CAD build for the part. Positions are in the model's coordinates, mm. A direction names the side the tool comes from. Give positions to 0.01 mm unless a question says otherwise; leave off trailing zeros. Loops run counter-clockwise (first coordinate to the right, second up) from the corner with the lowest first, then second, coordinate; pieces in that order, holes last. Notation, with made-up numbers: M 77.25,6.25 L 107.25,6.25 A17 cw 107.25,29.25 Z; hole C -12.75,40 d1. An arc over 180 degrees is marked long. Answer as CSV lines item,"result".
from build123d import *

# Parameters (mm, degrees)
BOSS_EXTRUDE1_DEPTH                               = 12.7
SKETCH2_R                                         = 4.1
CUT_EXTRUDE1_DEPTH                                = 51.982782527
CBORE_FOR_M5_HEX_HEAD_BOLT1_D                     = 2.5
CBORE_FOR_M5_HEX_HEAD_BOLT1_DEPTH                 = 18
CBORE_FOR_M5_HEX_HEAD_BOLT1_CBORE_D               = 5.6
CBORE_FOR_M5_HEX_HEAD_BOLT1_CBORE_DEPTH           = 2.7
CBORE_FOR_M5_HEX_HEAD_BOLT1_TIP                   = 0.751075774
CBORE_FOR_M5_HEX_HEAD_BOLT1_ON_FACE_2_D           = 2.5
CBORE_FOR_M5_HEX_HEAD_BOLT1_ON_FACE_2_DEPTH       = 18
CBORE_FOR_M5_HEX_HEAD_BOLT1_ON_FACE_2_CBORE_D     = 5.6
CBORE_FOR_M5_HEX_HEAD_BOLT1_ON_FACE_2_CBORE_DEPTH = 2.7
CBORE_FOR_M5_HEX_HEAD_BOLT1_ON_FACE_2_TIP         = 0.751075774


with BuildPart() as part:
    # Sketch1 → Boss-Extrude1 (new body)
    with BuildSketch(Plane(origin=(0, 0, 0), x_dir=(1, 0, 0), z_dir=(0, 1, 0))):
        with BuildLine():
            Line((-0.5, 37), (0.5, 37))
            ThreePointArc((0.5, 37), (2.621320344, 36.121320344), (3.5, 34))
            Line((3.5, 34), (3.5, 6.062177826))
            ThreePointArc((3.5, 6.062177826), (6.062177826, 3.5), (7, 0))
            Line((7, 0), (31.194863729, -13.968911087))
            ThreePointArc((31.194863729, -13.968911087), (32.592641208, -15.790530163), (32.29293994, -18.066987298))
            Line((32.29293994, -18.066987298), (31.79293994, -18.933012702))
            ThreePointArc((31.79293994, -18.933012702), (29.971320864, -20.330790181), (27.694863729, -20.031088913))
            Line((27.694863729, -20.031088913), (3.5, -6.062177826))
            ThreePointArc((3.5, -6.062177826), (0, -7), (-3.5, -6.062177826))
            Line((-3.5, -6.062177826), (-27.694863729, -20.031088913))
            ThreePointArc((-27.694863729, -20.031088913), (-29.971320864, -20.330790181), (-31.79293994, -18.933012702))
            Line((-31.79293994, -18.933012702), (-32.29293994, -18.066987298))
            ThreePointArc((-32.29293994, -18.066987298), (-32.592641208, -15.790530163), (-31.194863729, -13.968911087))
            Line((-31.194863729, -13.968911087), (-7, 0))
            ThreePointArc((-7, 0), (-6.062177826, 3.5), (-3.5, 6.062177826))
            Line((-3.5, 6.062177826), (-3.5, 34))
            ThreePointArc((-3.5, 34), (-2.621320344, 36.121320344), (-0.5, 37))
        make_face()
    extrude(amount=BOSS_EXTRUDE1_DEPTH)

    # Sketch2 → Cut-Extrude1 (cut, through all)
    with BuildSketch(Plane(origin=(0, 12.7, 0), x_dir=(1, 0, 0), z_dir=(0, 1, 0))):
        with Locations(Location((0, 0, 0), (0, 0, 270))):
            Circle(SKETCH2_R)
    extrude(amount=-CUT_EXTRUDE1_DEPTH, mode=Mode.SUBTRACT)

    # CBORE for M5 Hex Head Bolt1
    with Locations(Plane(origin=(-0.022879542, 6.389773721, 6.999962609), x_dir=(0.99999465842, 0, 0.003268506014), z_dir=(-0.003268506014, 0, 0.99999465842))):
        with Locations((0, 0)):
            CounterBoreHole(CBORE_FOR_M5_HEX_HEAD_BOLT1_D / 2, CBORE_FOR_M5_HEX_HEAD_BOLT1_CBORE_D / 2, CBORE_FOR_M5_HEX_HEAD_BOLT1_CBORE_DEPTH, depth=CBORE_FOR_M5_HEX_HEAD_BOLT1_DEPTH)
            with Locations((0, 0, -(CBORE_FOR_M5_HEX_HEAD_BOLT1_DEPTH + CBORE_FOR_M5_HEX_HEAD_BOLT1_TIP / 2))):  # 118° drill point
                Cone(0, CBORE_FOR_M5_HEX_HEAD_BOLT1_D / 2, CBORE_FOR_M5_HEX_HEAD_BOLT1_TIP, mode=Mode.SUBTRACT)

    # CBORE for M5 Hex Head Bolt1 on face 2
    with Locations(Plane(origin=(1.383929949, -4.684067914, 0), x_dir=(0.99999465842, 0, 0.003268506014), z_dir=(-0.003268506014, 0, 0.99999465842))):
        with Locations((0, 0)):
            CounterBoreHole(CBORE_FOR_M5_HEX_HEAD_BOLT1_ON_FACE_2_D / 2, CBORE_FOR_M5_HEX_HEAD_BOLT1_ON_FACE_2_CBORE_D / 2, CBORE_FOR_M5_HEX_HEAD_BOLT1_ON_FACE_2_CBORE_DEPTH, depth=CBORE_FOR_M5_HEX_HEAD_BOLT1_ON_FACE_2_DEPTH)
            with Locations((0, 0, -(CBORE_FOR_M5_HEX_HEAD_BOLT1_ON_FACE_2_DEPTH + CBORE_FOR_M5_HEX_HEAD_BOLT1_ON_FACE_2_TIP / 2))):  # 118° drill point
                Cone(0, CBORE_FOR_M5_HEX_HEAD_BOLT1_ON_FACE_2_D / 2, CBORE_FOR_M5_HEX_HEAD_BOLT1_ON_FACE_2_TIP, mode=Mode.SUBTRACT)


solid = part.part
1) Band-saw the part on C-C on z = -18. Give the cut face in (x, y).
Answer below:
outline,"M -3.5,0 L 3.5,0 L 3.5,12.7 L -3.5,12.7 Z"
2) Band-saw the part on B-B on z = 10.5. Give the cut face in (x, y).
Answer below:
outline,"M -25.19,0 L -11.19,0 L -11.19,12.7 L -25.19,12.7 Z; M 11.19,0 L 25.19,0 L 25.19,12.7 L 11.19,12.7 Z"
3) Band-saw the part on A-A on y = 2. Give the cut face in (x, z), and give its area (3 significant figures).
Answer below:
outline,"M -32.29,18.07 A3 ccw -31.19,13.97 L -7,0 A7 ccw -3.5,-6.06 L -3.5,-34 A3 ccw -0.5,-37 L 0.5,-37 A3 ccw 3.5,-34 L 3.5,-6.06 A7 ccw 7,0 L 31.19,13.97 A3 ccw 32.29,18.07 L 31.79,18.93 A3 ccw 27.69,20.03 L 3.5,6.06 A7 ccw -3.5,6.06 L -27.69,20.03 A3 ccw -31.79,18.93 Z; hole C 0,0 d8.2"
area,"726 mm^2"
4) Flat gauge pins, fed straight in: pin 1 (4 mm diameter, centred on y = 1.5, z = -5.5, fed in from +X); pin 2 (2 mm diameter, centred on y = 5, z = -27.5, fed in from -X); pin 3 (1 mm diameter, centred on x = -25.5, y = 6.5, fed in from -Z). Where does each tip first touch, or does it go through?
Answer below:
pin 1,"stops at x = 6.06"
pin 2,"stops at x = -3.5"
pin 3,"stops at z = 10.39"
5) Mould opens along Y. For faces 4 (the face through (0.2, 0, 4.3)), 5 (the face through (15.767, 6.261, 13.144)), 6 (the face through (0.155, 6.573, -11.62)) say: +Y half, -Y half, draft (parallel to the pull), parting line (faces both ways), or undercut.
Answer below:
face 4,"-Y half"
face 5,"draft"
face 6,"undercut"
6) Band-saw the part on D-D on x = 15. Give the cut face in (y, z).
Answer below:
outline,"M 0,4.62 L 12.7,4.62 L 12.7,12.7 L 0,12.7 Z"
7) Which spindle directions (+Z, -Z, +X, -X, +Y, -Y) get a long thin tool onto all of the face, cutting with end or side? Do faces 1 (the face through (-3.5, 6, -20)), 2 (the face through (-15.43, 6.26, 12.95)), 3 (the face through (18.93, 6.26, 6.89)). Say none if no direction does.
Answer below:
face 1,"-Z, -X, +Y, -Y"
face 2,"+Z, +Y, -Y"
face 3,"-Z, +X, +Y, -Y"
8) Drill centre lines: line 1 (X direction, y = 6.5, z = 0); line 2 (Z direction, x = 0, y = 8.25); line 3 (X direction, y = 11, z = -20.5). Where is each one in solid material? Low to high. Write a range as from..to.
Answer below:
line 1,"x = -7..-4.1, 4.1..7"
line 2,"z = -37..-4.1, 4.1..4.3"
line 3,"x = -3.5..3.5"
